Verification items for the finished model (mm, model axes). Round coordinates to 2 decimals unless told otherwise and drop trailing zeros. Write each loop counter-clockwise with the first axis right and the second up, starting at its lowest first coordinate (ties: lowest second). Pieces come first, ordered by that corner, then holes. Notation, with made-up numbers: (7.5, 65) - (25.5, 65) arc R27 ccw to (25.5, 85) - close; hole circle Ø4 at (-36, 70). An arc over 180 degrees is marked (long way). Answer as a JSON object with one key per item and string values.
```python
from build123d import *
from build123d.topology import SkipClean

# Parameters (mm, degrees)
SKETCH_1_R          = 1.5
SKETCH_1_R_2        = 5
EXTRUDE_1_DEPTH     = 3
SKETCH_2_R          = 57.5
SKETCH_2_R_2        = 55
EXTRUDE_2_DEPTH     = 25
EXTRUDE_START       = -3
SKETCH_3_R          = 1.5
EXTRUDE_3_DEPTH     = 3
CUT_EXTRUDE_START   = -30
SKETCH_4_R          = 69.475087651
SKETCH_4_R_2        = 57.5
CUT_EXTRUDE_1_DEPTH = 30
CUT_EXTRUDE_2_DEPTH = 10


with BuildPart() as part:
    # Sketch 1 → Extrude 1 (new body)
    with BuildSketch(Plane(origin=(0, 0, 0), x_dir=(1, 0, 0), z_dir=(0, 1, 0))):
        with BuildLine():
            Line((57.421685799, 3), (60, 3))
            ThreePointArc((60, 3), (63, 0), (60, -3))
            Line((60, -3), (57.421685799, -3))
            ThreePointArc((57.421685799, -3), (28.75, -49.796460718), (-26.112766688, -51.22863863))
            Line((-26.112766688, -51.22863863), (-27.401923789, -53.461524227))
            ThreePointArc((-27.401923789, -53.461524227), (-31.5, -54.559600438), (-32.598076211, -50.461524227))
            Line((-32.598076211, -50.461524227), (-31.308919111, -48.22863863))
            ThreePointArc((-31.308919111, -48.22863863), (-57.5, 0), (-31.308919111, 48.22863863))
            Line((-31.308919111, 48.22863863), (-32.598076211, 50.461524227))
            ThreePointArc((-32.598076211, 50.461524227), (-31.5, 54.559600438), (-27.401923789, 53.461524227))
            Line((-27.401923789, 53.461524227), (-26.112766688, 51.22863863))
            ThreePointArc((-26.112766688, 51.22863863), (28.75, 49.796460718), (57.421685799, 3))
        make_face()
        with Locations(Location((0, 8, 0), (0, 0, 270))):
            Circle(SKETCH_1_R, mode=Mode.SUBTRACT)
        with Locations(Location((8, 0, 0), (0, 0, 270))):
            Circle(SKETCH_1_R, mode=Mode.SUBTRACT)
        with Locations(Location((0, -8, 0), (0, 0, 270))):
            Circle(SKETCH_1_R, mode=Mode.SUBTRACT)
        with Locations(Location((-8, 0, 0), (0, 0, 270))):
            Circle(SKETCH_1_R, mode=Mode.SUBTRACT)
        with Locations(Location((0, 0, 0), (0, 0, 270))):
            Circle(SKETCH_1_R_2, mode=Mode.SUBTRACT)
        with Locations(Location((60, 0, 0), (0, 0, 270))):
            Circle(SKETCH_1_R, mode=Mode.SUBTRACT)
        with Locations(Location((-30, -51.961524227, 0), (0, 0, 270))):
            Circle(SKETCH_1_R, mode=Mode.SUBTRACT)
        with Locations(Location((-30, 51.961524227, 0), (0, 0, 270))):
            Circle(SKETCH_1_R, mode=Mode.SUBTRACT)
        with BuildLine():
            Line((10.583005244, 3), (29.849623113, 3))
            ThreePointArc((29.849623113, 3), (25.980762114, 15), (17.522887768, 24.350531909))
            Line((17.522887768, 24.350531909), (7.889578833, 7.66515139))
            ThreePointArc((7.889578833, 7.66515139), (9.526279442, 5.5), (10.583005244, 3))
        make_face(mode=Mode.SUBTRACT)
        with BuildLine():
            Line((10.583005244, -3), (29.849623113, -3))
            ThreePointArc((29.849623113, -3), (25.980762114, -15), (17.522887768, -24.350531909))
            Line((17.522887768, -24.350531909), (7.889578833, -7.66515139))
            ThreePointArc((7.889578833, -7.66515139), (9.526279442, -5.5), (10.583005244, -3))
        make_face(mode=Mode.SUBTRACT)
        with BuildLine():
            Line((2.693426411, -10.66515139), (12.326735345, -27.350531909))
            ThreePointArc((12.326735345, -27.350531909), (0, -30), (-12.326735345, -27.350531909))
            Line((-12.326735345, -27.350531909), (-2.693426411, -10.66515139))
            ThreePointArc((-2.693426411, -10.66515139), (0, -11), (2.693426411, -10.66515139))
        make_face(mode=Mode.SUBTRACT)
        with BuildLine():
            Line((-14.837519563, 31.699337741), (-24.860984224, 49.060487802))
            ThreePointArc((-24.860984224, 49.060487802), (0, 55), (24.860984224, 49.060487802))
            Line((24.860984224, 49.060487802), (14.837519563, 31.699337741))
            ThreePointArc((14.837519563, 31.699337741), (0, 35), (-14.837519563, 31.699337741))
        make_face(mode=Mode.SUBTRACT)
        with BuildLine():
            Line((-7.889578833, -7.66515139), (-17.522887768, -24.350531909))
            ThreePointArc((-17.522887768, -24.350531909), (-25.980762114, -15), (-29.849623113, -3))
            Line((-29.849623113, -3), (-10.583005244, -3))
            ThreePointArc((-10.583005244, -3), (-9.526279442, -5.5), (-7.889578833, -7.66515139))
        make_face(mode=Mode.SUBTRACT)
        with BuildLine():
            Line((-10.583005244, 3), (-29.849623113, 3))
            ThreePointArc((-29.849623113, 3), (-25.980762114, 15), (-17.522887768, 24.350531909))
            Line((-17.522887768, 24.350531909), (-7.889578833, 7.66515139))
            ThreePointArc((-7.889578833, 7.66515139), (-9.526279442, 5.5), (-10.583005244, 3))
        make_face(mode=Mode.SUBTRACT)
        with BuildLine():
            Line((20.033671986, 28.699337741), (30.057136647, 46.060487802))
            ThreePointArc((30.057136647, 46.060487802), (47.631397208, 27.5), (54.918120871, 3))
            Line((54.918120871, 3), (34.871191548, 3))
            ThreePointArc((34.871191548, 3), (30.310889132, 17.5), (20.033671986, 28.699337741))
        make_face(mode=Mode.SUBTRACT)
        with BuildLine():
            Line((-20.033671986, 28.699337741), (-30.057136647, 46.060487802))
            ThreePointArc((-30.057136647, 46.060487802), (-47.631397208, 27.5), (-54.918120871, 3))
            Line((-54.918120871, 3), (-34.871191548, 3))
            ThreePointArc((-34.871191548, 3), (-30.310889132, 17.5), (-20.033671986, 28.699337741))
        make_face(mode=Mode.SUBTRACT)
        with BuildLine():
            Line((-2.693426411, 10.66515139), (-12.326735345, 27.350531909))
            ThreePointArc((-12.326735345, 27.350531909), (0, 30), (12.326735345, 27.350531909))
            Line((12.326735345, 27.350531909), (2.693426411, 10.66515139))
            ThreePointArc((2.693426411, 10.66515139), (0, 11), (-2.693426411, 10.66515139))
        make_face(mode=Mode.SUBTRACT)
        with BuildLine():
            Line((-34.871191548, -3), (-54.918120871, -3))
            ThreePointArc((-54.918120871, -3), (-47.631397208, -27.5), (-30.057136647, -46.060487802))
            Line((-30.057136647, -46.060487802), (-20.033671986, -28.699337741))
            ThreePointArc((-20.033671986, -28.699337741), (-30.310889132, -17.5), (-34.871191548, -3))
        make_face(mode=Mode.SUBTRACT)
        with BuildLine():
            Line((34.871191548, -3), (54.918120871, -3))
            ThreePointArc((54.918120871, -3), (47.631397208, -27.5), (30.057136647, -46.060487802))
            Line((30.057136647, -46.060487802), (20.033671986, -28.699337741))
            ThreePointArc((20.033671986, -28.699337741), (30.310889132, -17.5), (34.871191548, -3))
        make_face(mode=Mode.SUBTRACT)
        with BuildLine():
            Line((14.837519563, -31.699337741), (24.860984224, -49.060487802))
            ThreePointArc((24.860984224, -49.060487802), (0, -55), (-24.860984224, -49.060487802))
            Line((-24.860984224, -49.060487802), (-14.837519563, -31.699337741))
            ThreePointArc((-14.837519563, -31.699337741), (0, -35), (14.837519563, -31.699337741))
        make_face(mode=Mode.SUBTRACT)
    extrude(amount=EXTRUDE_1_DEPTH)

    # Sketch 2 → Extrude 2 (add)
    with SkipClean():  # the faces are left unmerged after this step: merging them gives an invalid solid
        with BuildSketch(Plane(origin=(0, 3, 0), x_dir=(1, 0, 0), z_dir=(0, 1, 0))):
            with Locations(Location((0, 0, 0), (0, 0, 117.009297093))):
                Circle(SKETCH_2_R)
            with Locations(Location((0, 0, 0), (0, 0, 63.126776114))):
                Circle(SKETCH_2_R_2, mode=Mode.SUBTRACT)
        extrude(amount=EXTRUDE_2_DEPTH)

    # Sketch 3 → Extrude 3 (add)
    # profile 1 of 3: a face of its own
    with SkipClean():  # the faces are left unmerged after this step: merging them gives an invalid solid
        with BuildSketch(Plane(origin=(0, 28, 0), x_dir=(1, 0, 0), z_dir=(0, 1, 0)).offset(EXTRUDE_START)):
            with BuildLine():
                Line((-32.598076211, 50.461524227), (-31.308919111, 48.22863863))
                ThreePointArc((-31.308919111, 48.22863863), (-28.75, 49.796460718), (-26.112766688, 51.22863863))
                Line((-26.112766688, 51.22863863), (-27.401923789, 53.461524227))
                ThreePointArc((-27.401923789, 53.461524227), (-31.5, 54.559600438), (-32.598076211, 50.461524227))
            make_face()
            with Locations(Location((-30, 51.961524227, 0), (0, 0, 270))):
                Circle(SKETCH_3_R, mode=Mode.SUBTRACT)
        # profile 2 of 3: a face of its own
        with BuildSketch(Plane(origin=(0, 28, 0), x_dir=(1, 0, 0), z_dir=(0, 1, 0)).offset(EXTRUDE_START)):
            with BuildLine():
                Line((60, 3), (57.421685799, 3))
                ThreePointArc((57.421685799, 3), (57.5, 0), (57.421685799, -3))
                Line((57.421685799, -3), (60, -3))
                ThreePointArc((60, -3), (63, 0), (60, 3))
            make_face()
            with Locations(Location((60, 0, 0), (0, 0, 270))):
                Circle(SKETCH_3_R, mode=Mode.SUBTRACT)
        # profile 3 of 3: a face of its own
        with BuildSketch(Plane(origin=(0, 28, 0), x_dir=(1, 0, 0), z_dir=(0, 1, 0)).offset(EXTRUDE_START)):
            with BuildLine():
                Line((-27.401923789, -53.461524227), (-26.112766688, -51.22863863))
                ThreePointArc((-26.112766688, -51.22863863), (-28.75, -49.796460718), (-31.308919111, -48.22863863))
                Line((-31.308919111, -48.22863863), (-32.598076211, -50.461524227))
                ThreePointArc((-32.598076211, -50.461524227), (-31.5, -54.559600438), (-27.401923789, -53.461524227))
            make_face()
            with Locations(Location((-30, -51.961524227, 0), (0, 0, 270))):
                Circle(SKETCH_3_R, mode=Mode.SUBTRACT)
        extrude(amount=EXTRUDE_3_DEPTH)

    # Sketch 4 → Cut-Extrude 1 (cut)
    with SkipClean():  # the faces are left unmerged after this step: merging them gives an invalid solid
        with BuildSketch(Plane(origin=(0, 3, 0), x_dir=(1, 0, 0), z_dir=(0, 1, 0)).offset(CUT_EXTRUDE_START)):
            Circle(SKETCH_4_R)
            with Locations(Location((0, 0, 0), (0, 0, 117.009297093))):
                Circle(SKETCH_4_R_2, mode=Mode.SUBTRACT)
        extrude(amount=CUT_EXTRUDE_1_DEPTH, mode=Mode.SUBTRACT)
    add(part.part.scale(1), mode=Mode.REPLACE)  # the faces are merged on a copy

    # Sketch 5 → Cut-Extrude 2 (cut)
    with BuildSketch(Plane.XZ):
        Polygon((-20.031496469, -40.695569636), (-10.067965636, -23.43822801), (9.224847601, -21.977904737), (20.031496469, -40.695569636), align=None)
    extrude(amount=-CUT_EXTRUDE_2_DEPTH, mode=Mode.SUBTRACT)


solid = part.part
```
1. Cross-section at B-B (x = 0). Record the boundary of the cut face in (y, z).
Completed:
{"outline": "(0, -57.5) - (28, -57.5) - (28, -55) - (0, -55) - close; (0, -11) - (3, -11) - (3, -9.5) - (0, -9.5) - close; (0, -6.5) - (3, -6.5) - (3, -5) - (0, -5) - close; (0, 5) - (3, 5) - (3, 6.5) - (0, 6.5) - close; (0, 9.5) - (3, 9.5) - (3, 11) - (0, 11) - close; (0, 30) - (3, 30) - (3, 35) - (0, 35) - close; (0, 55) - (28, 55) - (28, 57.5) - (0, 57.5) - close"}
2. Cross-section at A-A (z = 0). Record the boundary of the cut face in (x, y), plus the area to 4 significant figures.
Completed:
{"outline": "(-57.5, 0) - (-9.5, 0) - (-9.5, 3) - (-55, 3) - (-55, 28) - (-57.5, 28) - close; (-6.5, 0) - (-5, 0) - (-5, 3) - (-6.5, 3) - close; (5, 0) - (6.5, 0) - (6.5, 3) - (5, 3) - close; (9.5, 0) - (57.5, 0) - (57.5, 25) - (58.5, 25) - (58.5, 28) - (55, 28) - (55, 3) - (9.5, 3) - close; (61.5, 25) - (63, 25) - (63, 28) - (61.5, 28) - close", "area": "429.5 mm^2"}
3. Cross-section at C-C (x = 50). Record the boundary of the cut face in (y, z).
Completed:
{"outline": "(0, -28.39) - (28, -28.39) - (28, -22.91) - (0, -22.91) - close; (0, -3) - (3, -3) - (3, 3) - (0, 3) - close; (0, 22.91) - (28, 22.91) - (28, 28.39) - (0, 28.39) - close"}
4. Material ranges on probe 1 along X at (y, z) = (1.85, 0); probe 2 along X at (y, z) = (26, 0); probe 3 along Z at (x, y) = (0, 12.25), recorded low to high. Write a range as from..to.
Completed:
{"probe 1": "x = -57.5..-9.5, -6.5..-5, 5..6.5, 9.5..57.5", "probe 2": "x = -57.5..-55, 55..58.5, 61.5..63", "probe 3": "z = -57.5..-55, 55..57.5"}
5. Go/stop test with flat-tipped pins: pin 1 (3.5 mm diameter, centred on x = -20, y = 1, fed in from +Z); pin 2 (6 mm diameter, centred on x = -31.5, y = 10.5, fed in from -Z); pin 3 (1 mm diameter, centred on y = 11.5, z = -18.5, fed in from +X); pin 4 (2.5 mm diameter, centred on x = 60, z = 0, fed in from +Y). Record where each tip stops, or that it passes through.
Completed:
{"pin 1": "stops at z = 54.53", "pin 2": "stops at z = -49.94", "pin 3": "stops at x = 54.61", "pin 4": "passes through"}
6. Cross-section at D-D (z = 39.5). Record the boundary of the cut face in (x, y).
Completed:
{"outline": "(-41.79, 0) - (-38.27, 0) - (-38.27, 28) - (-41.79, 28) - close; (-26.27, 0) - (-19.34, 0) - (-19.34, 3) - (-26.27, 3) - close; (19.34, 0) - (26.27, 0) - (26.27, 3) - (19.34, 3) - close; (38.27, 0) - (41.79, 0) - (41.79, 28) - (38.27, 28) - close"}
7. Mould release check, pull along X, two halves, no side actions. Record for faces 1 (the face through (0, 1, 30)), 2 (the face through (-28.8, 25, 50.8)): released by +X, released by -X, zero draft, split by the parting line, or undercut.
Completed:
{"face 1": "undercut", "face 2": "zero draft"}
